Here's how the part is built. I have some questions about the finished solid (model axes, mm). A direction names the side the tool comes from. Give positions to 0.01 mm unless a question says otherwise; leave off trailing zeros. Loops run counter-clockwise (first coordinate to the right, second up) from the corner with the lowest first, then second, coordinate; pieces in that order, holes last. Notation, with made-up numbers: (-38, 31) - (-13, 31) arc R21 cw to (-13, 50) - close; hole circle Ø4 at (-9, -12). An arc over 180 degrees is marked (long way). Return JSON: item names as keys, results as strings. Group by question number.
(1) On a 3-axis mill with a long thin cutter (end or side, diameter ignored), from which of +Z, -Z, +X, -X, +Y, -Y can I reach the whole of each face in a straight line? I mean faces 1 (the flat face through (1, 49, -18.755)), 2 (the cylindrical face through (89.194, 114.05, 58.235)), 3 (the flat face through (33, 0, 58)), 4 (the flat face through (3, 49, 20)), 5 (the flat face through (90, 35, 60)). Say none if no direction works.
(2) For P1, Ø10, axis at y = 84.5, z = 50, coming from the +X side; P2, Ø1.5, axis at x = 49, y = 76, coming from the -Z side; P3, Ø24, axis at x = 52.5, z = 36, coming from the +Y side, each with a flat end and sliding along its axis, tell me the tip position at first contact or that it passes through.
(3) If we section it at D-D (y = 118): Please give me the cut outline in (x, z).
(4) If we section it at B-B (z = -7): Please give me the cut outline in (x, y).
(5) If we section it at A-A (y = 47): Please give me the cut outline in (x, z) (3 decimals), then the cut area to 3 significant figures.
(6) I need wall thicknesses on probe 1 along Z at (x, y) = (90.5, 10); probe 2 along Z at (x, y) = (90, 18); probe 3 along Z at (x, y) = (21, 64.5). Which ranges of each line are inside material? Lowest first, please. Write a range as [from, to].
(7) If we mould it in two halves opening along X, with no side actions, what happens to faces 6 (the cylindrical face through (88.9, 17.26, 59.57)), 7 (the flat face through (33, 100, 58)), 8 (the flat face through (93, 49, 59))? For each: released by +X, released by -X, zero draft, split by the parting line, or undercut.
(8) If we section it at C-C (x = 46): Please give me the cut outline in (y, z).
Autodesk Fusion 360 part; units mm, degrees
sketch "스케치1" plane through (0, 0, 0) normal (0, 1, 0) x (1, 0, 0)
  line L0 (0, 0) -> (6, 0)
  line L1 (0, 0) -> (0, -62)
  line L2 (0, -62) -> (93, -62)
  line L3 (6, 0) -> (6, -57)
  line L4 (6, -57) -> (93, -57)
  line L5 (93, -57) -> (93, -62)
  line L6 (6, -57) -> (3, -57)
  line L7 (3, -57) -> (3, 0)
  line L8 (3, 0) -> (6, 0)
  line L9 (6, 0) -> (6, -57)
  dimension "d1" = 6
  dimension "d2" = 62
  dimension "d3" = 93
  dimension "d4" = 57
extrude "돌출1" add sketch "스케치1" along normal blind 100 contours L0 L1 L2 L4 L5 L6 L7
sketch "스케치2" plane through (0, 0, 0) normal (0, -1, 0) x (1, 0, 0)
  line L0 (0, 62) -> (0, 0)
  line L1 (0, 0) -> (3, 0)
  line L2 (3, 57) -> (93, 57)
  line L3 (93, 57) -> (93, 62)
  line L4 (93, 62) -> (0, 62)
  line L5 (93, 62) -> (88, 62)
  line L6 (88, 62) -> (88, 57)
  line L7 (88, 57) -> (93, 57)
  line L8 (93, 57) -> (93, 62)
  circle A0 centre (90.5, 59.5) radius 1.6
  line L9 (3, 0) -> (3, 57)
  dimension "d7" = 3.2
extrude "돌출2" cut sketch "스케치2" against normal blind 35 contours A0
sketch "스케치3" plane through (0, 100, 0) normal (0, 1, 0) x (-1, 0, 0)
  line L0 (0, 0) -> (0, 62)
  line L1 (0, 62) -> (-93, 62)
  line L2 (-93, 62) -> (-93, 57)
  line L3 (-93, 57) -> (-3, 57)
  line L4 (-3, 0) -> (0, 0)
  line L5 (-93, 62) -> (-87, 62)
  line L6 (-87, 62) -> (-87, 57)
  line L7 (-87, 57) -> (-93, 57)
  line L8 (-93, 57) -> (-93, 62)
  circle A0 centre (-90, 59.5) radius 1.5
  line L9 (-3, 57) -> (-3, 0)
  dimension "d10" = 3
extrude "돌출3" add sketch "스케치3" along normal blind 30 contours A0
fillet "필렛1" radius 1.5 1 edges at (91.3985, 130, 58.9576)
fillet "필렛2" radius 2.5 1 edges at (0, 50, 62)
extrude "돌출4" add 1 faces at (1, 66.6667, 0) along direction (0, 0, -1) blind 18.755
Values:
{
 "1": {"face 1": "-Z, +X, -X, +Y, -Y", "face 2": "+Y", "face 3": "+Z, -Z, +X, -X, -Y", "face 4": "-Z, +X, +Y, -Y", "face 5": "-Y"},
 "2": {"P1": "x = 3", "P2": "z = 57", "P3": "through"},
 "3": {"outline": "circle Ø3 at (90, 59.5)"},
 "4": {"outline": "(0, 0) - (3, 0) - (3, 100) - (0, 100) - close"},
 "5": {"outline": "(0, -18.755) - (3, -18.755) - (3, 57) - (93, 57) - (93, 62) - (2.5, 62) arc R2.5 ccw to (0, 59.5) - close", "area": "691 mm2"},
 "6": {"probe 1": "[57, 57.9], [61.1, 62]", "probe 2": "[57, 57.98], [61.02, 62]", "probe 3": "[57, 62]"},
 "7": {"face 6": "undercut", "face 7": "zero draft", "face 8": "released by +X"},
 "8": {"outline": "(0, 57) - (100, 57) - (100, 62) - (0, 62) - close"}
}
